Part print with two shaded views. Sizes in mm from the minimum x, y, z corner. A direction names the side the tool comes from. Coordinates: 2 decimals unless noted, no trailing zeros. Write each loop counter-clockwise with the first axis right and the second up, starting at its lowest first coordinate (ties: lowest second). Pieces come first, ordered by that corner, then holes. Notation, with made-up numbers: (54.25, 66.25) - (107.25, 66.25) arc R24 ccw to (107.25, 103.25) - close; hole circle Ø7 at (-2.5, 52.5). An arc over 180 degrees is marked (long way). Answer in a Markdown table with one row per item. Add a question column.
Q1. Band-saw the part on D-D (x = 10). List the corners of the cut face in (y, z).
Q2. Two-plate mould, pull along X, no slides. Class the marked faces 4, 5 and 6: +X half, -X half, draft (parallel to the pull), parting line (faces both ways), or undercut.
Q3. Band-saw the part on A-A (x = 3.9). List the corners of the cut face in (y, z).
Q4. Drill centre lines: line 1 along Y through (x, z) = (3.9, 10.8); line 2 along Z through (x, y) = (7, 5.75); line 3 along Z through (x, y) = (30, 4). Where is each one in solid material? Low to high. Write a range as from..to.
Q5. 3-axis set-ups, long thin cutter, end or side, ignore diameter. For the marked faces 1, 2 and 3: which of +Z, -Z, +X, -X, +Y, -Y reach the whole face in a straight line?
Q6. Pin check, flat tips, straight feed: pin 1 (4 mm diameter, centred on x = 25, y = 4.5, fed in from -Z); pin 2 (1.5 mm diameter, centred on x = 27.5, y = 3, fed in from +Z); pin 3 (2.5 mm diameter, centred on x = 23.5, y = 5, fed in from -Z). Stop position of each tip, or through.
Q7. Band-saw the part on C-C (z = 5.75). List the corners of the cut face in (x, y), and give its area (3 significant figures).
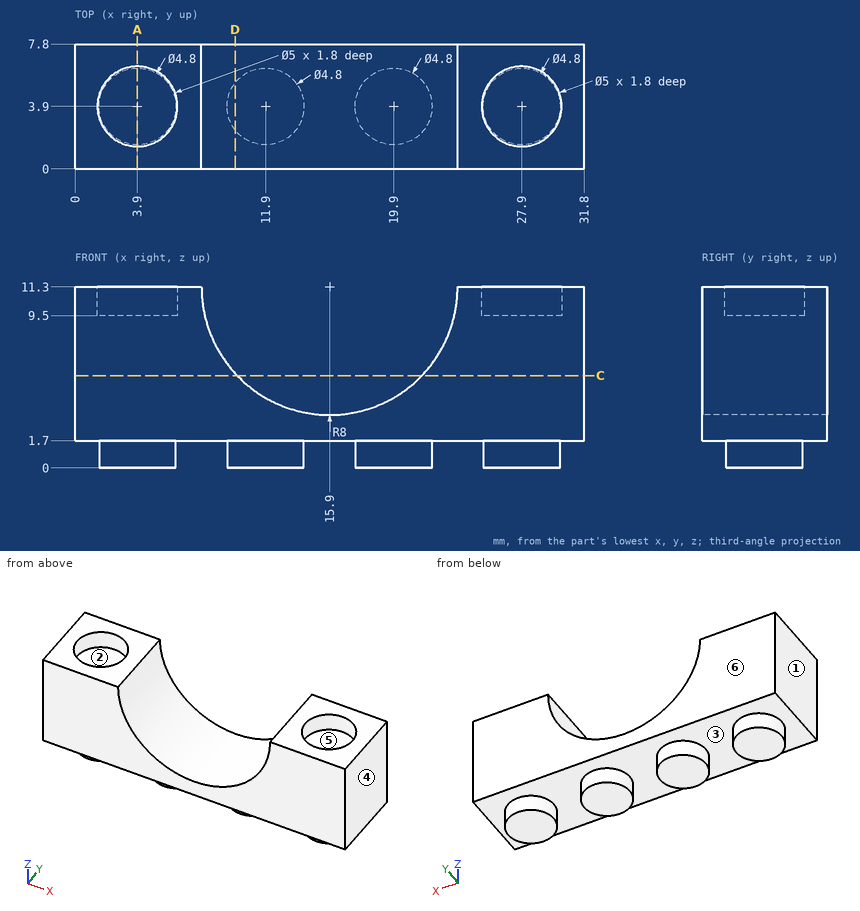
Checked values:
| question | item | result |
|---|---|---|
| 1 | outline | (0, 1.7) - (2.43, 1.7) - (2.43, 0) - (5.37, 0) - (5.37, 1.7) - (7.8, 1.7) - (7.8, 5.9) - (0, 5.9) - close |
| 2 | face 4 | +X half |
| 2 | face 5 | undercut |
| 2 | face 6 | draft |
| 3 | outline | (0, 1.7) - (1.5, 1.7) - (1.5, 0) - (6.3, 0) - (6.3, 1.7) - (7.8, 1.7) - (7.8, 11.3) - (6.4, 11.3) - (6.4, 9.5) - (1.4, 9.5) - (1.4, 11.3) - (0, 11.3) - close |
| 4 | line 1 | y = 0..1.4, 6.4..7.8 |
| 4 | line 2 | z = 1.7..11.3 |
| 4 | line 3 | z = 0..9.5 |
| 5 | face 1 | +Z, -Z, -X, +Y, -Y |
| 5 | face 2 | +Z |
| 5 | face 3 | -Z |
| 6 | pin 1 | stops at z = 0 |
| 6 | pin 2 | stops at z = 9.5 |
| 6 | pin 3 | stops at z = 1.7 |
| 7 | outline | (0, 0) - (10.14, 0) - (10.14, 7.8) - (0, 7.8) - close; (21.66, 0) - (31.8, 0) - (31.8, 7.8) - (21.66, 7.8) - close |
| 7 | area | 158 mm² |
